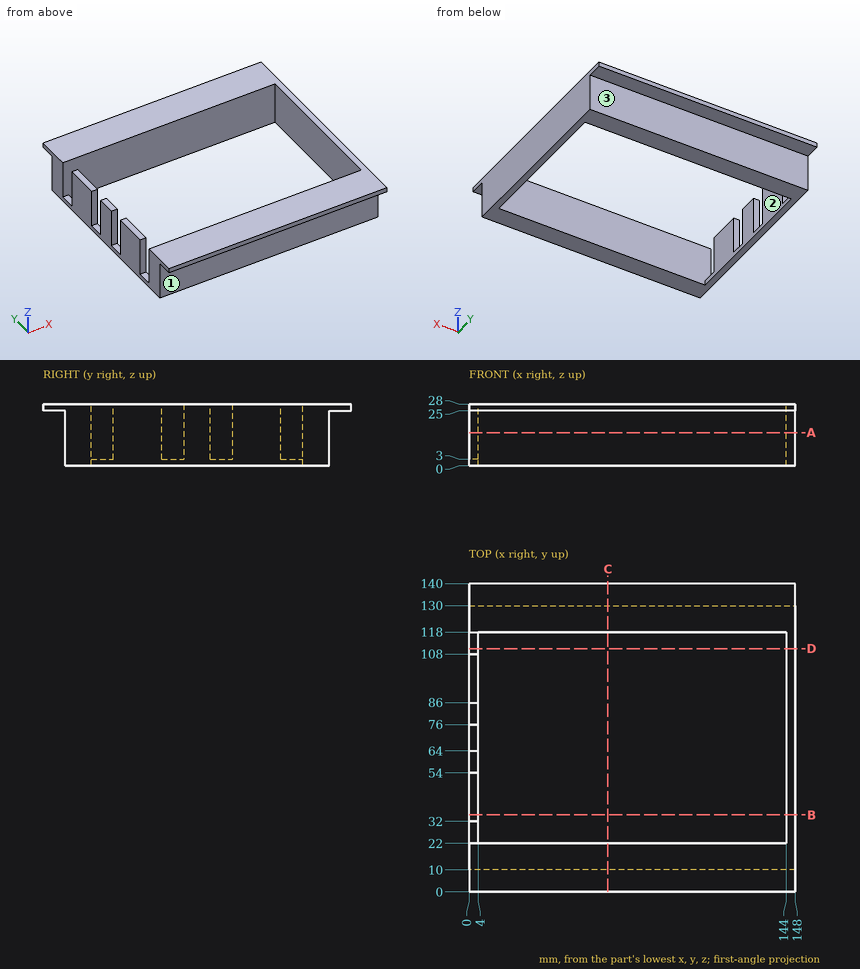
The drawing under review shows one solid part. Ordinate dimensions are in mm from its lowest x, y, z. A direction names the side the tool comes from. Round coordinates to 2 decimals unless told otherwise and drop trailing zeros. Write each loop counter-clockwise with the first axis right and the second up, starting at its lowest first coordinate (ties: lowest second). Pieces come first, ordered by that corner, then holes. Notation, with made-up numbers: (60.25, 11) - (100.25, 11) arc R11 cw to (100.25, 22) - close; hole circle Ø10 at (70.5, -10). An arc over 180 degrees is marked (long way). Use a Markdown table: item, result. Add a question column.
1. Clearance check with flat-ended pins moving along their axes: pin 1 (1.5 mm diameter, centred on y = 102, z = 25, fed in from -X); pin 2 (2 mm diameter, centred on x = 1.5, y = 113.5, fed in from +Z); pin 3 (4.5 mm diameter, centred on x = 1.5, z = 14.5, fed in from +Y); pin 4 (1.2 mm diameter, centred on x = 2, z = 17.5, fed in from -Y). State where each tip first meets the part, or that it passes through.
2. Wall thickness on probe 1 along X at (y, z) = (43.5, 3); probe 2 along Y at (x, z) = (55.5, 3.5); probe 3 along X at (y, z) = (79, 13.5): over which ranges is each line inside the solid? List them lowest first.
3. We need section C-C (x = 63). State the section outline as (y, z) points, then the cut area to 3 significant figures.
4. We need section D-D (y = 110.5). State the section outline as (x, z) points, then the cut area to 3 significant figures.
5. For the marked faces 1, 2 and 3, list the 3-axis set-ups (+Z, -Z, +X, -X, +Y, -Y) from which the entire face can be reached by the end or side of a thin tool; tool diameter is ignored.
6. We need section A-A (z = 15). State the section outline as (x, y) points, then the cut area to 3 significant figures.
7. We need section B-B (y = 35). State the section outline as (x, z) points.
Output:
| question | item | result |
|---|---|---|
| 1 | pin 1 | stops at x = 0 |
| 1 | pin 2 | stops at z = 3 |
| 1 | pin 3 | stops at y = 130 |
| 1 | pin 4 | stops at y = 10 |
| 2 | probe 1 | x = 0 to 4, 144 to 148 |
| 2 | probe 2 | y = 10 to 22, 118 to 130 |
| 2 | probe 3 | x = 144 to 148 |
| 3 | outline | (0, 25) - (10, 25) - (10, 0) - (22, 0) - (22, 28) - (0, 28) - close; (118, 0) - (130, 0) - (130, 25) - (140, 25) - (140, 28) - (118, 28) - close |
| 3 | area | 732 mm2 |
| 4 | outline | (0, 0) - (4, 0) - (4, 3) - (0, 3) - close; (144, 0) - (148, 0) - (148, 28) - (144, 28) - close |
| 4 | area | 124 mm2 |
| 5 | face 1 | -Z, +X, -X, -Y |
| 5 | face 2 | +Z, -Z |
| 5 | face 3 | -Z, +X, -X, +Y |
| 6 | outline | (0, 10) - (148, 10) - (148, 130) - (0, 130) - (0, 118) - (144, 118) - (144, 22) - (0, 22) - close; (0, 32) - (4, 32) - (4, 54) - (0, 54) - close; (0, 64) - (4, 64) - (4, 76) - (0, 76) - close; (0, 86) - (4, 86) - (4, 108) - (0, 108) - close |
| 6 | area | 4,160 mm2 |
| 7 | outline | (0, 0) - (4, 0) - (4, 28) - (0, 28) - close; (144, 0) - (148, 0) - (148, 28) - (144, 28) - close |
